from build123d import *

# Parameters (mm, degrees)
HOLE_WIZARD_12_1_D       = 5.7912
PATTERN_CIRCULAR_1_COUNT = 4


with BuildPart() as part:
    # Model → Revolve 1 (revolve)
    with BuildSketch(Plane.XY, mode=Mode.PRIVATE) as revolve_1_sk:
        with BuildLine():
            Line((8.11136174, 12.552108092), (8.11136174, 17.150272129))
            Line((8.11136174, 17.150272129), (23.557930854, 17.150272129))
            Line((23.557930854, 17.150272129), (23.557930854, 22.076877203))
            Line((23.557930854, 22.076877203), (52.479166263, 22.076877203))
            Line((52.479166263, 22.076877203), (52.479166263, 23.062198021))
            Line((52.479166263, 23.062198021), (57.737573082, 23.062198021))
            Line((57.737573082, 23.062198021), (57.737573082, 25.410254309))
            Line((57.737573082, 25.410254309), (10.493573082, 25.410254309))
            ThreePointArc((10.493573082, 25.410254309), (8.809095288, 26.107987857), (8.11136174, 27.792465651))
            Line((8.11136174, 27.792465651), (8.11136174, 50.026438172))
            Line((8.11136174, 50.026438172), (7.317291293, 50.820508619))
            Line((7.317291293, 50.820508619), (4.141009504, 50.820508619))
            Line((4.141009504, 50.820508619), (3.346939057, 50.026438172))
            Line((3.346939057, 50.026438172), (3.346939057, 17.150272129))
            Line((3.346939057, 17.150272129), (8.11136174, 12.552108092))
        make_face()
    revolve(revolve_1_sk.sketch.rotate(Axis((0, 0, 0), (1, 0, 0)), 90), axis=Axis((0, 0, 0), (1, 0, 0)))

    # Hole Wizard 12 _1 (through all)
    with Locations(Plane.ZY.offset(-3.346939057)):
        with Locations((0, 33.02)):
            hole_wizard_12_1 = Hole(HOLE_WIZARD_12_1_D / 2)

    # Pattern Circular 1: Hole Wizard 12 _1 ×4 about axis
    pattern_circular_1_axis = Axis((0, 0, 0), (1, 0, 0))
    for i in range(1, PATTERN_CIRCULAR_1_COUNT):
        add(hole_wizard_12_1.rotate(pattern_circular_1_axis, i * 360 / PATTERN_CIRCULAR_1_COUNT), mode=Mode.SUBTRACT)


solid = part.part
Here's how the part is built. I have some questions about the finished solid (model axes, mm). A direction names the side the tool comes from. Give positions to 0.01 mm unless a question says otherwise; leave off trailing zeros. Order: outer loops, then holes, each group sorted by start corner. A loop starts at its lowest first (then second) coordinate and runs counter-clockwise, first axis right, second up. Notation, with made-up numbers: M -19.75,81 L 1.25,81 A8 ccw 1.25,91 Z; hole C 62,12.5 d9. An arc over 180 degrees is marked long. Answer as a JSON object with one key per item and string values. Group by question number.
1) I'm going to push flat-ended pins straight in: pin 1 Ø1 at (x, y) = (21, 7) entering from -Z; pin 2 Ø7.5 at (y, z) = (33.02, 0) entering from +X; pin 3 Ø8 at (x, z) = (19, 23) entering from +Y; pin 4 Ø5 at (y, z) = (2.5, 16) entering from -X. Where does each tip first touch, or does it pass through?
2) We'd pull the mould along Z, two halves only. Please class faces 3 (the flat face through (3.347, 22, -1)), 4 (the cylindrical face through (5.76, 0.38, -35.89)), 5 (the flat face through (52.479, 12, -19)), 6 (the cylindrical face through (5.707, -50.388, -6.616)): pulls with the +Z half, pulls with the -Z half, needs draft (parallel to the pull), parting line crosses it, or undercut.
3) Please list where these lines run through material, in increasing order: L1, parallel to Y at x = 6.25, z = 0; L2, parallel to Y at x = 37.5, z = 0.5; L3, parallel to Y at x = 4.55, z = 0. Write a range as [from, to].
4) On a 3-axis mill with a long thin cutter (end or side, diameter ignored), from which of +Z, -Z, +X, -X, +Y, -Y can I reach the whole of each face in a straight line? I mean faces 1 (the cylindrical face through (5.76, -0.38, 35.89)), 2 (the cylindrical face through (15.94, -14.46, 9.22)). Say none if no direction works.
5) Suppose I cut it at B-B, the plane z = 0. Count the separate pieces of the cut face and the enclosed holes in it, plus the area to 3 significant figures.
6) Suppose I cut it at A-A, the plane x = 39. Write out the boundary of the cut face in (y, z), plus the area to 3 significant figures.
Results found:
{
 "1": {"pin 1": "z = -24.56", "pin 2": "x = 8.11", "pin 3": "y = 16.87", "pin 4": "x = 3.35"},
 "2": {"face 3": "needs draft", "face 4": "undercut", "face 5": "undercut", "face 6": "parting line crosses it"},
 "3": {"L1": "[-50.82, -35.92], [-30.12, -14.35], [14.35, 30.12], [35.92, 50.82]", "L2": "[-25.41, -22.07], [22.07, 25.41]", "L3": "[-50.82, -35.92], [-30.12, -15.99], [15.99, 30.12], [35.92, 50.82]"},
 "4": {"face 1": "+X, -X", "face 2": "+X"},
 "5": {"separate pieces": "4", "enclosed holes": "0", "area": "761 mm²"},
 "6": {"outline": "C 0,0 d50.82; hole C 0,0 d44.15", "area": "497 mm²"}
}
